Can you work these out from the model? Positions are in its coordinate system, mm. A direction names the side the tool comes from. Give positions to 0.01 mm unless a question says otherwise; leave off trailing zeros. Order: outer loops, then holes, each group sorted by start corner. A loop starts at its lowest first (then second) coordinate and runs counter-clockwise, first axis right, second up. Notation, with made-up numbers: (-22, 22) - (-2, 22) arc R18 cw to (-2, 42) - close; hole circle Ø1 at (-4.75, 75.25). An arc over 180 degrees is marked (long way). Answer as CSV lines item,"result".
Autodesk Inventor part; units mm, degrees
ref_plane "YZ Plane" through (0, 0, 0) normal (1, 0, 0) x (0, 1, 0)
ref_plane "XZ Plane" through (0, 0, 0) normal (0, 1, 0) x (-1, 0, 0)
ref_plane "XY Plane" through (0, 0, 0) normal (0, 0, 1) x (1, 0, 0)
sketch "草圖1" plane through (0, 0, 0) normal (0, 0, 1) x (1, 0, 0)
  line L0 (-6.2319, 0) -> (37.3914, 0) construction
  line L1 (0, -62.7215) -> (0, 388.8794) construction
  line L2 (0, 324.365) -> (31.1595, 324.365)
  line L3 (31.1595, 324.365) -> (31.1595, 65.285)
  line L4 (31.1595, 65.285) -> (0, 65.285)
  line L5 (0, 65.285) -> (0, 324.365)
  line L6 (0, 65.285) -> (18.4838, 65.285)
  line L7 (18.4838, 65.285) -> (18.4838, 1.7929)
  line L8 (18.4838, 1.7929) -> (0, 1.7929)
  line L9 (0, 1.7929) -> (0, 65.285)
  line L10 (31.1595, 306.585) -> (30.6515, 306.585)
  line L11 (30.6515, 306.585) -> (30.6515, 263.405)
  line L12 (30.6515, 263.405) -> (31.1595, 263.405)
  line L13 (31.1595, 263.405) -> (31.1595, 306.585)
  line L14 (31.1595, 250.705) -> (30.6515, 250.705)
  line L15 (30.6515, 250.705) -> (30.6515, 207.525)
  line L16 (30.6515, 207.525) -> (31.1595, 207.525)
  line L17 (31.1595, 207.525) -> (31.1595, 250.705)
  line L18 (31.1595, 194.825) -> (30.6515, 194.825)
  line L19 (30.6515, 194.825) -> (30.6515, 151.645)
  line L20 (30.6515, 151.645) -> (31.1595, 151.645)
  line L21 (31.1595, 151.645) -> (31.1595, 194.825)
  line L22 (31.1595, 138.945) -> (30.6515, 138.945)
  line L23 (30.6515, 138.945) -> (30.6515, 65.285)
  line L24 (30.6515, 65.285) -> (31.1595, 65.285)
  line L25 (31.1595, 65.285) -> (31.1595, 138.945)
  point P0 (31.1595, 151.645)
  point P1 (31.1595, 207.525)
  point P2 (31.1595, 263.405)
  dimension "d7" = 0.508
  dimension "d8" = 43.18
  dimension "d9" = 43.18
  dimension "d10" = 17.78
  dimension "d11" = 12.7
  dimension "d12" = 12.7
  dimension "d13" = 43.18
  dimension "d18" = 12.7
revolve "迴轉1" add sketch "草圖1" angle 360 about axis through (0, 65.285, 0) along (0, 1, 0)
sketch "草圖2" plane through (0, 0, 0) normal (0, 1, 0) x (-1, 0, 0)
  line L0 (38.1, -38.1) -> (-38.1, -38.1)
  line L1 (-38.1, -38.1) -> (-38.1, 38.1)
  line L2 (-38.1, 38.1) -> (38.1, 38.1)
  line L3 (38.1, 38.1) -> (38.1, -38.1)
  line L4 (53.34, 0) -> (-53.34, 0) construction
  line L5 (0, -53.34) -> (0, 53.34) construction
  point P0 (0, 0)
  dimension "d5" = 76.2
  dimension "d6" = 76.2
extrude "擠出1" add sketch "草圖2" along normal blind 14.2875
revolve "迴轉2" cut sketch "草圖1" angle 360 about axis through (0, -10, 0) along (0, 1, 0) contours L3 L12 L11 L10 | L23 L22 L3 L4 | L3 L16 L15 L14 | L3 L20 L19 L18
fillet "圓角1" radius 5.08 1 edges at (-31.1595, 324.365, 0)
fillet "圓角2" radius 7.62 1 edges at (-18.4838, 14.2875, 0)
fillet "圓角3" radius 3.175 4 edges at (38.1, 14.2875, 0) (-38.1, 14.2875, 0) (0, 14.2875, 38.1) (0, 14.2875, -38.1)
properties part number "警示燈"
1) If we mould it in two halves opening along Y, with no side actions, what happens to faces 1 (the flat face through (1, 0, 1)), 2 (the flat face through (1, 5, 38.1)), 3 (the flat face through (13.2, 65.285, 13.2))? For each: +Y half, -Y half, draft (parallel to the pull), parting line (faces both ways), or undercut.
Answer block:
face 1,"-Y half"
face 2,"draft"
face 3,"undercut"
2) I need wall thicknesses on line 1 along Y through (x, z) = (15.5, 22) (1 decimal); line 2 along Y through (x, z) = (24.5, 15) (1 decimal); line 3 along Y through (x, z) = (-31, -29). Which ranges of each line are inside material? Lowest first, please. Write a range as [from, to].
Answer block:
line 1,"[0, 14.3], [65.3, 324.3]"
line 2,"[0, 14.3], [65.3, 323.6]"
line 3,"[0, 14.29]"
3) I'm going to push flat-ended pins straight in: P1, Ø5, axis at y = 76, z = 6.5, coming from the +X side; P2, Ø8, axis at x = 0, y = 53.5, coming from the +Z side; P3, Ø1, axis at y = 176.5, z = -9.5, coming from the +X side. Where does each tip first touch, or does it pass through?
Answer block:
P1,"x = 30.39"
P2,"z = 18.48"
P3,"x = 29.3"
4) Which directions (+Z, -Z, +X, -X, +Y, -Y) give clear straight access to the entire face, cutting with the end or side of a thin tool? Please do faces 4 (the flat face through (38.1, 5, -1)), 5 (the flat face through (22.9, 207.525, 20.6)), 6 (the cylindrical face through (29.72, 312.85, 9.36)).
Answer block:
face 4,"+Z, -Z, +X, +Y, -Y"
face 5,"none"
face 6,"+Y"
5) I want a section at A-A on y = 181. Write out the boundary of the cut face in (x, z), plus the area to 3 significant figures.
Answer block:
outline,"circle Ø61.3 at (0, 0)"
area,"2,950 mm2"
6) I want a section at B-B on y = 38.5. Write out the boundary of the cut face in (x, z).
Answer block:
outline,"circle Ø36.97 at (0, 0)"
